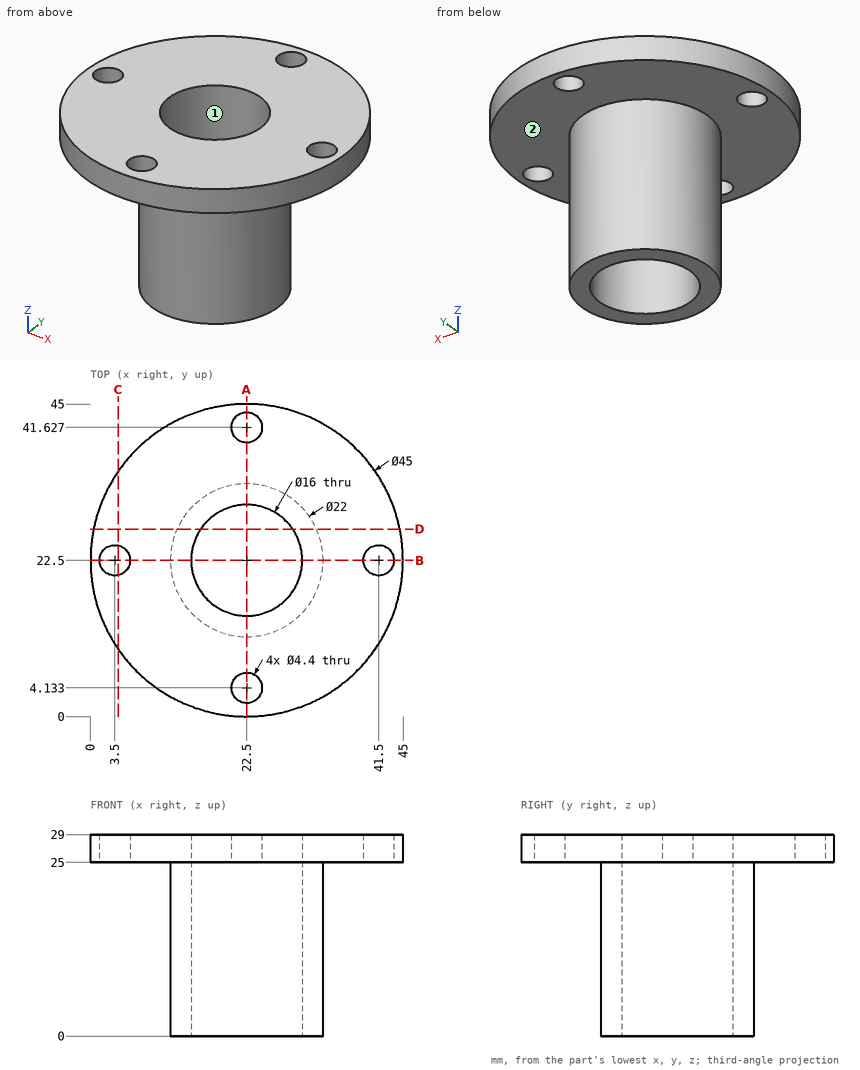
The figure shows three views and two pictorial views of one solid part (mm, origin at its lowest corner). Answer the questions. A direction names the side the tool comes from. Coordinates: 2 decimals unless noted, no trailing zeros. Loops run counter-clockwise (first coordinate to the right, second up) from the corner with the lowest first, then second, coordinate; pieces in that order, holes last.
(1) The part is cut by section C-C (x = 4). Determine the outline of the cut face in (y, z).
Solution:
outline: (9.69, 25) - (20.36, 25) - (20.36, 29) - (9.69, 29) - close; (24.64, 25) - (35.31, 25) - (35.31, 29) - (24.64, 29) - close
(2) The part is cut by section A-A (x = 22.5). Determine the outline of the cut face in (y, z), and give its area (3 significant figures).
Solution:
outline: (0, 25) - (1.93, 25) - (1.93, 29) - (0, 29) - close; (6.33, 25) - (11.5, 25) - (11.5, 0) - (14.5, 0) - (14.5, 29) - (6.33, 29) - close; (30.5, 0) - (33.5, 0) - (33.5, 25) - (39.43, 25) - (39.43, 29) - (30.5, 29) - close; (43.83, 25) - (45, 25) - (45, 29) - (43.83, 29) - close
area: 231 mm2
(3) A tool of negligible diameter and unlimited length cuts with its end or side. For the marked faces 1 and 2, from which of +Z, -Z, +X, -X, +Y, -Y can it reach the whole face along a straight path? Write none if from no direction.
Solution:
face 1: +Z, -Z
face 2: -Z
(4) Flat-ended cylindrical pins translate along their axes: pin 1 Ø2 at (x, y) = (22, 9.5) entering from -Z; pin 2 Ø2.5 at (x, y) = (3.5, 22.5) entering from -Z; pin 3 Ø18.5 at (x, y) = (22.5, 22.5) entering from +Z; pin 4 Ø1.5 at (y, z) = (27, 21.5) entering from +X. Find the tip coordinate at first contact, or state that the pin passes through.
Solution:
pin 1: stops at z = 25
pin 2: passes through
pin 3: stops at z = 29
pin 4: stops at x = 32.84
(5) The part is cut by section B-B (y = 22.5). Determine the outline of the cut face in (x, z).
Solution:
outline: (0, 25) - (1.3, 25) - (1.3, 29) - (0, 29) - close; (5.7, 25) - (11.5, 25) - (11.5, 0) - (14.5, 0) - (14.5, 29) - (5.7, 29) - close; (30.5, 0) - (33.5, 0) - (33.5, 25) - (39.3, 25) - (39.3, 29) - (30.5, 29) - close; (43.7, 25) - (45, 25) - (45, 29) - (43.7, 29) - close
(6) The part is cut by section D-D (y = 27). Determine the outline of the cut face in (x, z) (1 decimal).
Solution:
outline: (0.5, 25) - (12.5, 25) - (12.5, 0) - (15.9, 0) - (15.9, 29) - (0.5, 29) - close; (29.1, 0) - (32.5, 0) - (32.5, 25) - (44.5, 25) - (44.5, 29) - (29.1, 29) - close
(7) Consider line 1 along Y through (x, z) = (22.5, 27.85); line 2 along Y through (x, z) = (22.5, 15); line 3 along Z through (x, y) = (7.5, 36). Determine where each line is inside the solid, lowest interval first.
Solution:
line 1: y = 0 to 1.93, 6.33 to 14.5, 30.5 to 39.43, 43.83 to 45
line 2: y = 11.5 to 14.5, 30.5 to 33.5
line 3: z = 25 to 29
